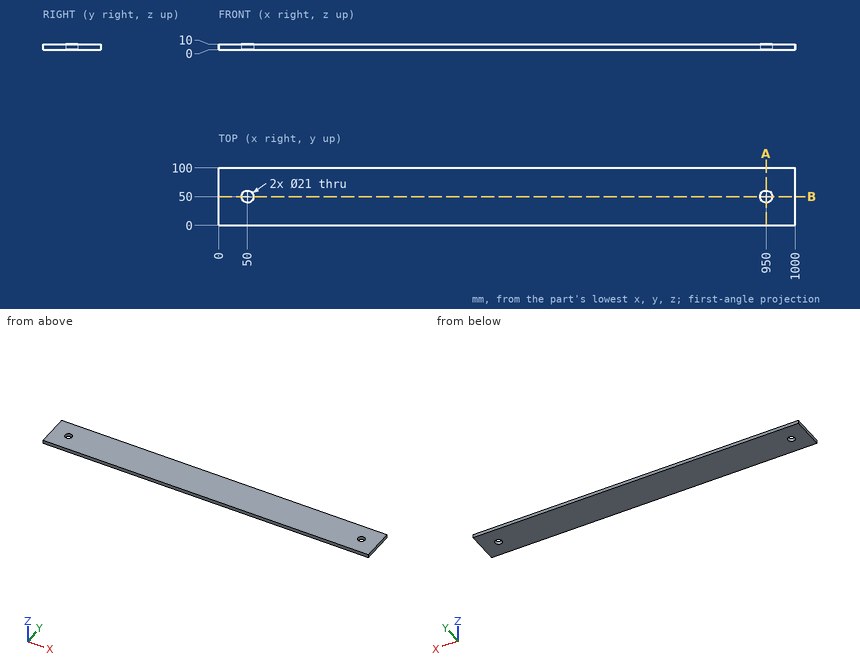
Here's the drawing with two shaded views (mm, measured from the low corner). I have some questions. Give positions to 0.01 mm unless a question says otherwise; leave off trailing zeros. Order: outer loops, then holes, each group sorted by start corner. A loop starts at its lowest first (then second) coordinate and runs counter-clockwise, first axis right, second up. Notation, with made-up numbers: (19, 88) -> (58, 88) arc R28 ccw to (58, 108) -> close; hole circle Ø6 at (-32.5, 44). An arc over 180 degrees is marked (long way). Use a Markdown table: item, result. Add a question column.
Item 1: Imagine slicing it at B-B on y = 50. Please give me the cut outline in (x, z).
Item 2: Imagine slicing it at A-A on x = 950. Please give me the cut outline in (y, z).
Item 3: I need wall thicknesses on line 1 (Y direction, x = 950, z = 7.75); line 2 (X direction, y = 41.5, z = 6.25); line 3 (X direction, y = 42, z = 2.25). Which ranges of each line are inside material? Lowest first, please.
Item 4: Will this pin go through, and if not, where does the flat tip stop? pin 1 (17 mm diameter, centred on x = 50, y = 50, fed in from +Z).
Data:
| question | item | result |
|---|---|---|
| 1 | outline | (0, 0) -> (39.5, 0) -> (39.5, 10) -> (0, 10) -> close; (60.5, 0) -> (939.5, 0) -> (939.5, 10) -> (60.5, 10) -> close; (960.5, 0) -> (1000, 0) -> (1000, 10) -> (960.5, 10) -> close |
| 2 | outline | (0, 0) -> (39.5, 0) -> (39.5, 10) -> (0, 10) -> close; (60.5, 0) -> (100, 0) -> (100, 10) -> (60.5, 10) -> close |
| 3 | line 1 | y = 0 to 39.5, 60.5 to 100 |
| 3 | line 2 | x = 0 to 43.84, 56.16 to 943.84, 956.16 to 1000 |
| 3 | line 3 | x = 0 to 43.2, 56.8 to 943.2, 956.8 to 1000 |
| 4 | pin 1 | passes through |
